Source: CAD feature listing. Evaluate the final solid. Frame: model axes, mm. A direction names the side the tool comes from. Round coordinates to 2 decimals unless told otherwise and drop trailing zeros. Loops run counter-clockwise (first coordinate to the right, second up) from the corner with the lowest first, then second, coordinate; pieces in that order, holes last. Notation, with made-up numbers: M 24.25,73.5 L 42.25,73.5 A34 ccw 42.25,109.5 Z; hole C 27,36.25 d3. An arc over 180 degrees is marked long. Write each question's results on one line, items separated by ' | '. Start each with the question number.
1. Section A-A on y = -26.5. Output: boundary loops of the cut face in (x, z).
2. Section C-C on y = -68. Output: boundary loops of the cut face in (x, z).
3. Contact query for flat-ended pins moving along their axis: pin 1 Ø1.5 at (y, z) = (-78.5, 4.5) entering from -X; pin 2 Ø4 at (y, z) = (35.5, -4.5) entering from +X; pin 3 Ø3.5 at (y, z) = (-76.5, -3.5) entering from +X; pin 4 Ø2.5 at (x, y) = (-164, -26.5) entering from +Z. Output: stop coordinate, or through.
4. Section B-B on z = -8. Give the number of separate pieces and of enclosed holes in the cut face, and give its area (3 significant figures).
5. Draft query along Y for faces 6 (the flat face through (-119, 83.15, 0)), 7 (the flat face through (-125.05, -77, 0)), 8 (the flat face through (-119, -83.15, 0)). Return one class per face: released by +Y, released by -Y, zero draft, split by the parting line, or undercut.
6. Section D-D on y = 65. Output: boundary loops of the cut face in (x, z).
7. Ray query, line 1 (Y direction, x = -117, z = 19); line 2 (Y direction, x = -164, z = -7); line 3 (Y direction, x = -127, z = -22.5). Return the intervals inside material, ascending.
8. Set-up query: faces 1 (the flat face through (-128, 79, 0)), 2 (the flat face through (-157, 27, 0)), 3 (the cylindrical face through (-162.6, -27.784, 0.418)), 4 (the flat face through (-128, -79, 0)), 5 (the flat face through (-169.989, 0, 0)). Return all of +Z, -Z, +X, -X, +Y, -Y with unobstructed straight access to the full face (end or side cutting, diameter ignored); none if empty.
from build123d import *

# Parameters (mm, degrees)
EXTRUDE_START       = -29.85
EXTRUDE_1_DEPTH     = 59.7
CUT_EXTRUDE_START   = 30.35
SKETCH_2_R          = 1.9
CUT_EXTRUDE_1_DEPTH = 60.7


with BuildPart() as part:
    # 草图1 → 凸台-拉伸1 (new body)
    with BuildSketch(Plane.XY.offset(EXTRUDE_START)):
        with BuildLine():
            Line((-111.7, 80.15), (-123.55, 80.15))
            ThreePointArc((-123.55, 80.15), (-124.257106781, 79.857106781), (-124.55, 79.15))
            Line((-124.55, 79.15), (-124.55, 75.550213562))
            ThreePointArc((-124.55, 75.550213562), (-124.626120467, 75.16753013), (-124.842893219, 74.843106781))
            Line((-124.842893219, 74.843106781), (-126.773, 72.913))
            Line((-126.773, 72.913), (-160.353049521, 34.659710148))
            ThreePointArc((-160.353049521, 34.659710148), (-160.512493197, 33.587513726), (-159.601529381, 33))
            Line((-159.601529381, 33), (-159, 33))
            ThreePointArc((-159, 33), (-157.585786438, 32.414213562), (-157, 31))
            Line((-157, 31), (-157, 23.5))
            ThreePointArc((-157, 23.5), (-158.171572875, 20.671572875), (-161, 19.5))
            Line((-161, 19.5), (-162.989, 19.5))
            ThreePointArc((-162.989, 19.5), (-165.817427125, 18.328427125), (-166.989, 15.5))
            Line((-166.989, 15.5), (-166.989, -15.5))
            ThreePointArc((-166.989, -15.5), (-165.817427125, -18.328427125), (-162.989, -19.5))
            Line((-162.989, -19.5), (-161, -19.5))
            ThreePointArc((-161, -19.5), (-158.171572875, -20.671572875), (-157, -23.5))
            Line((-157, -23.5), (-157, -31))
            ThreePointArc((-157, -31), (-157.585786438, -32.414213562), (-159, -33))
            Line((-159, -33), (-159.601529381, -33))
            ThreePointArc((-159.601529381, -33), (-160.512493197, -33.587513726), (-160.353049521, -34.659710148))
            Line((-160.353049521, -34.659710148), (-126.773, -72.913))
            Line((-126.773, -72.913), (-125.342893219, -74.343106781))
            ThreePointArc((-125.342893219, -74.343106781), (-125.126120467, -74.66753013), (-125.05, -75.050213562))
            Line((-125.05, -75.050213562), (-125.05, -79.15))
            ThreePointArc((-125.05, -79.15), (-124.757106781, -79.857106781), (-124.05, -80.15))
            Line((-124.05, -80.15), (-111.7, -80.15))
            ThreePointArc((-111.7, -80.15), (-110.851471863, -80.501471863), (-110.5, -81.35))
            Line((-110.5, -81.35), (-110.5, -81.95))
            ThreePointArc((-110.5, -81.95), (-110.851471863, -82.798528137), (-111.7, -83.15))
            Line((-111.7, -83.15), (-126.5, -83.15))
            ThreePointArc((-126.5, -83.15), (-127.560660172, -82.710660172), (-128, -81.65))
            Line((-128, -81.65), (-128, -76.550320344))
            ThreePointArc((-128, -76.550320344), (-128.114180701, -75.976295195), (-128.439339828, -75.489660172))
            Line((-128.439339828, -75.489660172), (-128.963, -74.966))
            Line((-128.963, -74.966), (-165.023, -33.887))
            ThreePointArc((-165.023, -33.887), (-168.70682882, -27.745711718), (-169.989, -20.7))
            Line((-169.989, -20.7), (-169.989, 20.7))
            ThreePointArc((-169.989, 20.7), (-168.70682882, 27.745711718), (-165.023, 33.887))
            Line((-165.023, 33.887), (-128.963, 74.966))
            Line((-128.963, 74.966), (-128.439339828, 75.489660172))
            ThreePointArc((-128.439339828, 75.489660172), (-128.114180701, 75.976295195), (-128, 76.550320344))
            Line((-128, 76.550320344), (-128, 81.65))
            ThreePointArc((-128, 81.65), (-127.560660172, 82.710660172), (-126.5, 83.15))
            Line((-126.5, 83.15), (-111.7, 83.15))
            ThreePointArc((-111.7, 83.15), (-110.851471863, 82.798528137), (-110.5, 81.95))
            Line((-110.5, 81.95), (-110.5, 81.35))
            ThreePointArc((-110.5, 81.35), (-110.851471863, 80.501471863), (-111.7, 80.15))
        make_face()
    extrude(amount=EXTRUDE_1_DEPTH)

    # 草图2 → 切除-拉伸1 (cut)
    with BuildSketch(Plane.XY.offset(CUT_EXTRUDE_START)):
        with Locations(Location((-164, 26.5, 0), (0, 0, 180))):
            Circle(SKETCH_2_R)
        with Locations(Location((-164, -26.5, 0), (0, 0, 180))):
            Circle(SKETCH_2_R)
    extrude(amount=-CUT_EXTRUDE_1_DEPTH, mode=Mode.SUBTRACT)


solid = part.part
Taken from the geometry:
1) outline: M -169.13,-29.85 L -165.9,-29.85 L -165.9,29.85 L -169.13,29.85 Z; M -162.1,-29.85 L -157,-29.85 L -157,29.85 L -162.1,29.85 Z
2) outline: M -135.08,-29.85 L -131.09,-29.85 L -131.09,29.85 L -135.08,29.85 Z
3) pin 1: x = -128 | pin 2: x = -157.86 | pin 3: x = -125.05 | pin 4: through
4) separate pieces: 1 | enclosed holes: 2 | area: 885 mm^2
5) face 6: released by +Y | face 7: undercut | face 8: released by -Y
6) outline: M -137.71,-29.85 L -133.72,-29.85 L -133.72,29.85 L -137.71,29.85 Z
7) line 1: -83.15 to -80.15, 80.15 to 83.15 | line 2: -35.05 to -28.4, -24.6 to -19.37, 19.37 to 24.6, 28.4 to 35.05 | line 3: -83.06 to -72.65, 72.65 to 83.06
8) face 1: +Z, -Z, -X, +Y | face 2: +Z, -Z, +X | face 3: +Z, -Z | face 4: +Z, -Z, -X, -Y | face 5: +Z, -Z, -X, +Y, -Y
